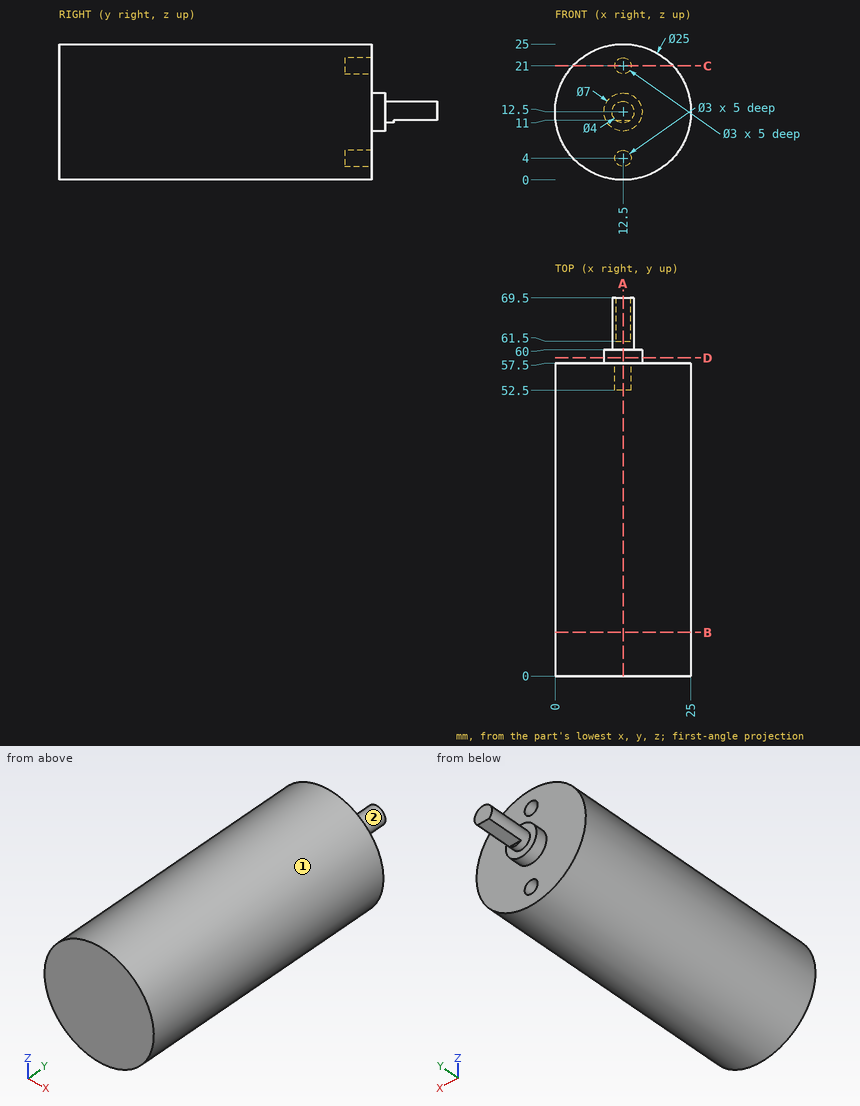
Verification items for this drawing (mm, ordinates from the low corner). A direction names the side the tool comes from. Give positions to 0.01 mm unless a question says otherwise; leave off trailing zeros. Write each loop counter-clockwise with the first axis right and the second up, starting at its lowest first coordinate (ties: lowest second). Pieces come first, ordered by that corner, then holes.
1) Cross-section at D-D (y = 58.5). Record the boundary of the cut face in (x, z).
Values follow:
outline: circle Ø7 at (12.5, 12.5)
2) Set-up check for the marked faces 1 and 2: record each of +Z, -Z, +X, -X, +Y, -Y from which the full face is reachable in a straight line by a thin tool's end or side.
Values follow:
face 1: +Y, -Y
face 2: +Y
3) Go/stop test with flat-tipped pins: pin 1 Ø1 at (y, z) = (28.5, 6.5) entering from -X (3 decimals); pin 2 Ø12.5 at (x, z) = (12, 14.5) entering from +Y; pin 3 Ø5 at (x, y) = (20.5, 48) entering from +Z (3 decimals); pin 4 Ø4 at (x, z) = (12.5, 21) entering from +Y. Record where each tip stops, or that it passes through.
Values follow:
pin 1: stops at x = 1.275
pin 2: stops at y = 69.5
pin 3: stops at z = 23.725
pin 4: stops at y = 57.5
4) Cross-section at B-B (y = 8). Record the boundary of the cut face in (x, z).
Values follow:
outline: circle Ø25 at (12.5, 12.5)
5) Cross-section at C-C (z = 21). Record the boundary of the cut face in (x, y), plus the area to 3 significant figures.
Values follow:
outline: (3.33, 0) - (21.67, 0) - (21.67, 57.5) - (14, 57.5) - (14, 52.5) - (11, 52.5) - (11, 57.5) - (3.33, 57.5) - close
area: 1,040 mm2
6) Cross-section at A-A (x = 12.5). Record the boundary of the cut face in (y, z).
Values follow:
outline: (0, 0) - (57.5, 0) - (57.5, 2.5) - (52.5, 2.5) - (52.5, 5.5) - (57.5, 5.5) - (57.5, 9) - (60, 9) - (60, 10.5) - (61.5, 10.5) - (61.5, 11) - (69.5, 11) - (69.5, 14.5) - (60, 14.5) - (60, 16) - (57.5, 16) - (57.5, 19.5) - (52.5, 19.5) - (52.5, 22.5) - (57.5, 22.5) - (57.5, 25) - (0, 25) - close
7) Thickness scan on line 1 (Y direction, x = 8.5, z = 21.75); line 2 (X direction, y = 55.3, z = 21); line 3 (Z direction, x = 16.75, y = 14). Record the ranges inside material, lowest first.
Values follow:
line 1: y = 0 to 57.5
line 2: x = 3.33 to 11, 14 to 21.67
line 3: z = 0.74 to 24.26
